from build123d import *

# Parameters (mm, degrees)
SKETCH_1_R          = 1.25
SKETCH_1_R_2        = 1
EXTRUDE_1_DEPTH     = 2
CUT_EXTRUDE_1_DEPTH = 2


with BuildPart() as part:
    # 草圖1 → 填料-伸長1 (new body)
    with BuildSketch(Plane.XY):
        with BuildLine():
            Line((-17.216213198, 10.1625), (13.283786802, 10.1625))
            Line((13.283786802, 10.1625), (13.283786802, -21.8375))
            Line((13.283786802, -21.8375), (-17.216213198, -21.8375))
            Line((-17.216213198, -21.8375), (-19.716213198, -21.8375))
            Line((-19.716213198, -21.8375), (-25.716213198, -21.8375))
            Line((-25.716213198, -21.8375), (-25.716213198, -15.8375))
            ThreePointArc((-25.716213198, -15.8375), (-24.716213198, -14.8375), (-25.716213198, -13.8375))
            Line((-25.716213198, -13.8375), (-27.716213198, -13.8375))
            Line((-27.716213198, -13.8375), (-27.716213198, -9.8375))
            Line((-27.716213198, -9.8375), (-25.716213198, -9.8375))
            ThreePointArc((-25.716213198, -9.8375), (-24.716213198, -8.8375), (-25.716213198, -7.8375))
            Line((-25.716213198, -7.8375), (-25.716213198, -3.8375))
            ThreePointArc((-25.716213198, -3.8375), (-24.716213198, -2.8375), (-25.716213198, -1.8375))
            Line((-25.716213198, -1.8375), (-27.716213198, -1.8375))
            Line((-27.716213198, -1.8375), (-27.716213198, 2.1625))
            Line((-27.716213198, 2.1625), (-25.716213198, 2.1625))
            ThreePointArc((-25.716213198, 2.1625), (-24.716213198, 3.1625), (-25.716213198, 4.1625))
            Line((-25.716213198, 4.1625), (-25.716213198, 10.1625))
            Line((-25.716213198, 10.1625), (-21.716213198, 10.1625))
            Line((-21.716213198, 10.1625), (-17.216213198, 10.1625))
        make_face()
        with Locations((-19.216213198, 7.6625)):
            Circle(SKETCH_1_R, mode=Mode.SUBTRACT)
        with Locations((-19.216213198, -19.3375)):
            Circle(SKETCH_1_R, mode=Mode.SUBTRACT)
        with Locations((10.783786802, -19.3375)):
            Circle(SKETCH_1_R, mode=Mode.SUBTRACT)
        with Locations((10.783786802, 7.6625)):
            Circle(SKETCH_1_R, mode=Mode.SUBTRACT)
        with Locations((-23.716213198, 0.1625)):
            Circle(SKETCH_1_R_2, mode=Mode.SUBTRACT)
        with Locations((-23.716213198, -11.8375)):
            Circle(SKETCH_1_R_2, mode=Mode.SUBTRACT)
    extrude(amount=EXTRUDE_1_DEPTH)

    # 草圖4 → 除料-伸長1 (cut)
    with BuildSketch(Plane(origin=(0, 0, 0), x_dir=(-1, 0, 0), z_dir=(0, 0, -1))):
        with BuildLine():
            Line((-13.283786802, 5.1625), (-13.283786802, -16.8375))
            ThreePointArc((-13.283786802, -16.8375), (-2.283786802, -5.8375), (-13.283786802, 5.1625))
        make_face()
    extrude(amount=-CUT_EXTRUDE_1_DEPTH, mode=Mode.SUBTRACT)


solid = part.part
Input: part model. Units: mm. Frame: model coordinates. A direction names the side the tool comes from. Coordinates: 2 decimals unless noted, no trailing zeros. Loops run counter-clockwise (first coordinate to the right, second up) from the corner with the lowest first, then second, coordinate; pieces in that order, holes last. Notation, with made-up numbers: (81, 45) -> (102, 45) arc R17 ccw to (102, 64) -> close; hole circle Ø7 at (-14.75, 88). An arc over 180 degrees is marked (long way). Write each question's results on one line, items separated by ' | '. Start each with the question number.
Q1. Pull-direction query (Y, two-part tool) for faces 1 (the cylindrical face through (-22.76, 0.46, 0.99)), 2 (the flat face through (13.284, -19, 1)), 3 (the flat face through (-6, 10.162, 1)); classes: released by +Y, released by -Y, zero draft, split by the parting line, or undercut.
Q2. Section A-A, the plane z = 0.9. Return the cut outline in (x, y).
Q3. Section B-B, the plane y = -8.5. Return the cut outline in (x, z), plus the area to 3 significant figures.
Q4. Pin query (flat end, axial travel): pin 1 (1 mm diameter, centred on x = -26.5, z = 0.5, fed in from +Y); pin 2 (1 mm diameter, centred on y = -17.5, z = 1.5, fed in from -X); pin 3 (2 mm diameter, centred on x = 10.78, y = -19.34, fed in from -Z); pin 4 (1 mm diameter, centred on x = -26.5, z = 1.5, fed in from -Y). Return the tip coordinate at first contact, or that it passes through.
Q5. Reachability of faces 4 (the flat face through (-25.716, -19, 1)), 5 (the flat face through (-25.716, 7, 1)), 6 (the flat face through (-25.716, -6, 1)), 7 (the cylindrical face through (-19.4, -18.1, 1)) from +Z, -Z, +X, -X, +Y, -Y: full face, straight path, thin tool, end or side. Return the list, or none.
Q6. Ray query, line 1 (X direction, y = 7.5, z = 0.15); line 2 (Y direction, x = -25.5, z = 0.9); line 3 (X direction, y = 6, z = 0.8). Return the intervals inside material, ascending. Write a range as from..to.
Found:
1) face 1: undercut | face 2: zero draft | face 3: released by +Y
2) outline: (-27.72, -13.84) -> (-25.72, -13.84) arc R1 cw to (-25.72, -15.84) -> (-25.72, -21.84) -> (13.28, -21.84) -> (13.28, -16.84) arc R11 cw to (13.28, 5.16) -> (13.28, 10.16) -> (-25.72, 10.16) -> (-25.72, 4.16) arc R1 cw to (-25.72, 2.16) -> (-27.72, 2.16) -> (-27.72, -1.84) -> (-25.72, -1.84) arc R1 cw to (-25.72, -3.84) -> (-25.72, -7.84) arc R1 cw to (-25.72, -9.84) -> (-27.72, -9.84) -> close; hole circle Ø2 at (-23.72, -11.84); hole circle Ø2 at (-23.72, 0.16); hole circle Ø2.5 at (-19.22, -19.34); hole circle Ø2.5 at (-19.22, 7.66); hole circle Ø2.5 at (10.78, -19.34); hole circle Ø2.5 at (10.78, 7.66)
3) outline: (-24.77, 0) -> (2.61, 0) -> (2.61, 2) -> (-24.77, 2) -> close | area: 54.8 mm2
4) pin 1: y = 2.16 | pin 2: x = -25.72 | pin 3: through | pin 4: y = -13.84
5) face 4: +Z, -Z, -X, -Y | face 5: +Z, -Z, -X, +Y | face 6: +Z, -Z, -X | face 7: +Z, -Z
6) line 1: -25.72..-20.46, -17.98..9.54, 12.02..13.28 | line 2: -21.84..-15.81, -13.86..-9.81, -7.86..-3.81, -1.86..2.19, 4.14..10.16 | line 3: -25.72..13.28
